Autodesk Fusion 360 part; units mm, degrees
sketch "Sketch1" plane through (0, 0, 0) normal (0, 0, 1) x (1, 0, 0)
  line L0 (0, 0) -> (800, 0)
  line L1 (800, 0) -> (800, 400)
  line L2 (800, 400) -> (0, 400)
  line L3 (0, 400) -> (0, 0)
  dimension "d1" = 800
  dimension "d2" = 400
extrude "Extrude1" add sketch "Sketch1" along normal blind 90
sketch "Sketch2" plane through (0, 0, 0) normal (-1, 0, 0) x (0, -1, 0)
  line L0 (-400, 0) -> (0, 0)
  line L1 (0, 0) -> (0, 90)
  line L2 (0, 90) -> (-400, 90)
  line L3 (-400, 90) -> (-400, 0)
  line L4 (-200, 90) -> (-200, 60) construction
  line L5 (-200, 60) -> (-200, 30) construction
  line L6 (-200, 30) -> (-200, 0) construction
  line L7 (-400, 90) -> (0, 90) construction
  line L8 (0, 90) -> (0, 60) construction
  line L9 (0, 60) -> (-400, 60)
  line L10 (-400, 60) -> (-400, 90) construction
  line L11 (-400, 60) -> (0, 60) construction
  line L12 (0, 60) -> (0, 30) construction
  line L13 (0, 30) -> (-400, 30)
  line L14 (-400, 30) -> (-400, 60) construction
  dimension "d5" = 30
  dimension "d6" = 30
extrude "Extrude2" cut sketch "Sketch2" against normal blind 400 contours L1 L2 L3 L9
extrude "Extrude3" cut sketch "Sketch2" against normal blind 200 contours L1 L3 L9 L13
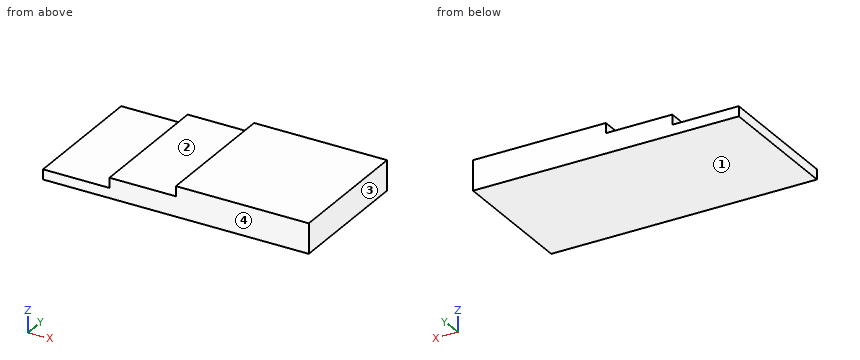
Could you check a few things on this model? Use its own coordinates, in mm. Face numbers are marked on the shaded views. A direction names the side the tool comes from. Round coordinates to 2 decimals unless told otherwise and drop trailing zeros. Write each loop counter-clockwise with the first axis right and the second up, starting at its lowest first coordinate (ties: lowest second). Pieces come first, ordered by that corner, then holes. Notation, with made-up numbers: (89, 74.25) - (129, 74.25) arc R24 ccw to (129, 112.25) - close; hole circle Ø2 at (-30.75, 51). An arc over 180 degrees is marked (long way). Use a Markdown table: item, result.
Q1. Please list where these lines run through material, in increasing order: L1, parallel to Z at x = 191, y = 52.5; L2, parallel to X at y = 223.5, z = 34.5; L3, parallel to Z at x = 355.5, y = 106.5.
Output values:
| item | result |
|---|---|
| L1 | 0 to 30 |
| L2 | 200 to 800 |
| L3 | 0 to 60 |
Q2. For the marked faces 1 and 2, which set-ups out of +Z, -Z, +X, -X, +Y, -Y let a thin tool reach every point of the face, with its end or its side?
Output values:
| item | result |
|---|---|
| face 1 | -Z, +X, -X, +Y, -Y |
| face 2 | +Z, -X, +Y, -Y |
Q3. For pin 1 (1 mm diameter, centred on x = 409, z = 42.5, fed in from -Y); pin 2 (24 mm diameter, centred on y = 189, z = 52.5, fed in from -X), each with a flat end and sliding along its axis, tell me the tip position at first contact or that it passes through.
Output values:
| item | result |
|---|---|
| pin 1 | y = 0 |
| pin 2 | x = 200 |
Q4. I want a section at C-C (x = 325.5). List the corners of the cut face in (y, z) for me.
Output values:
| item | result |
|---|---|
| outline | (0, 0) - (400, 0) - (400, 60) - (0, 60) - close |
Q5. Thinking about a two-plate mould opening in X: for the marked faces 3 and 4, which applies, released by +X, released by -X, zero draft, split by the parting line, or undercut?
Output values:
| item | result |
|---|---|
| face 3 | released by +X |
| face 4 | zero draft |
Q6. I want a section at A-A (y = 376). List the corners of the cut face in (x, z) for me.
Output values:
| item | result |
|---|---|
| outline | (0, 0) - (800, 0) - (800, 90) - (400, 90) - (400, 60) - (200, 60) - (200, 30) - (0, 30) - close |
Q7. I want a section at B-B (z = 76). List the corners of the cut face in (x, y) for me.
Output values:
| item | result |
|---|---|
| outline | (400, 0) - (800, 0) - (800, 400) - (400, 400) - close |
